Design review of the part built by this model. Coordinates are the model's own, in mm. Face numbers are marked on the shaded views. A direction names the side the tool comes from. Give positions to 0.01 mm unless a question says otherwise; leave off trailing zeros. Loops run counter-clockwise (first coordinate to the right, second up) from the corner with the lowest first, then second, coordinate; pieces in that order, holes last.
from build123d import *

# Parameters (mm, degrees)
SKETCH030_W             = 25
SKETCH030_H             = 15
PAD007_DEPTH            = 2
PAD008_DEPTH            = 7.5
SKETCH032_R             = 1.5
POCKET007_DEPTH         = 7.25
SKETCH031_R             = 1.75
POCKET008_DEPTH         = 5
PAD009_DEPTH            = 2
CHAMFER005_SIZE         = 1
SKETCH035_R             = 2.125
SKETCH035_R_2           = 1.75
PAD010_DEPTH            = 1.1
BODY003_PLACEMENT_ANGLE = 180


with BuildPart() as part:
    # Sketch030 → Pad007 (new body)
    with BuildSketch(Plane.YZ):
        Rectangle(SKETCH030_W, SKETCH030_H)
    extrude(amount=PAD007_DEPTH)

    # Sketch033 (on Face4 of Pad007) → Pad008 (join)
    with BuildSketch(Plane(origin=(0, 0, 7.5), x_dir=(0, -1, 0), z_dir=(0, 0, 1))):
        Polygon((-15, -23.23103), (15, -23.23103), (17, -9.88), (15, 2), (-15, 2), (-17, -9.88), align=None)
    extrude(amount=PAD008_DEPTH)

    # Sketch032 (on Face13 of Pad008) → Pocket007 (cut)
    with BuildSketch(Plane(origin=(0, 0, 15), x_dir=(0, -1, 0), z_dir=(0, 0, 1))):
        with Locations((11.75, -2.18)):
            Circle(SKETCH032_R)
        with Locations((-11.75, -2.18)):
            Circle(SKETCH032_R)
    extrude(amount=-POCKET007_DEPTH, mode=Mode.SUBTRACT)

    # Sketch031 (on Face4 of Pad008) → Pocket008 (cut)
    with BuildSketch(Plane(origin=(0, 0, 0), x_dir=(0, 1, 0), z_dir=(-1, 0, 0))):
        with Locations((-6.925, 0)):
            Circle(SKETCH031_R)
        with Locations((6.925, 0)):
            Circle(SKETCH031_R)
    extrude(amount=-POCKET008_DEPTH, mode=Mode.SUBTRACT)

    # Sketch034 (on Face1 of Pocket008) → Pad009 (join)
    with BuildSketch(Plane(origin=(0, -12.5, 0), x_dir=(0, 0, -1), z_dir=(0, -1, 0))):
        Polygon((-7.5, -9.88), (7.5, 0), (-7.5, 0), align=None)
    pad009 = extrude(amount=-PAD009_DEPTH)

    # Mirrored001: Pad009 across XZ
    add(pad009.mirror(Plane.XZ))

    # Chamfer005
    chamfer005_edges = [part.edges().sort_by_distance(p)[0] for p in [
        (-2.18, 13.25, 15),
        (-2.18, -10.25, 15),
    ]]
    chamfer(chamfer005_edges, length=CHAMFER005_SIZE)

    # Sketch035 (on Face19 of Chamfer005) → Pad010 (join, symmetric)
    with BuildSketch(Plane(origin=(1, 0, 0), x_dir=(0, 1, 0), z_dir=(-1, 0, 0))):
        with Locations((-6.925, 0)):
            Circle(SKETCH035_R)
        with Locations((-6.925, 0)):
            Circle(SKETCH035_R_2, mode=Mode.SUBTRACT)
        with Locations((6.925, 0)):
            Circle(SKETCH035_R)
        with Locations((6.925, 0)):
            Circle(SKETCH035_R_2, mode=Mode.SUBTRACT)
    extrude(amount=PAD010_DEPTH, both=True)


with BuildPart() as part_1:
    # Body003 placement: moved
    add(part.part.rotate(Axis((0, 0, 0), (1, 0, 0)), BODY003_PLACEMENT_ANGLE))


solid = part_1.part
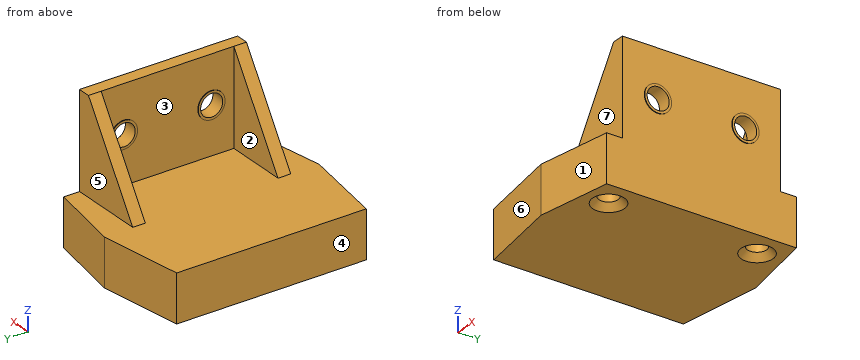
Q1. Tool access review of the marked faces 5, 6 and 7: name each direction out of +Z, -Z, +X, -X, +Y, -Y from which nothing blocks a thin tool from reaching the whole face with its end or side.
Results:
face 5: +Z, +X, -X, +Y
face 6: +Z, -Z, -X, -Y
face 7: +Z, +X, -X, -Y
Q2. Draft analysis for pull direction Y (two halves, no side actions). For the marked faces 1, 2, 3 and 4, state which applies: pulls with the +Y half, pulls with the -Y half, needs draft (parallel to the pull), parting line crosses it, or undercut.
Results:
face 1: pulls with the -Y half
face 2: undercut
face 3: undercut
face 4: needs draft
Q3. Take a section at B-B (z = 0). Give the number of separate pieces and of enclosed holes in the cut face, plus the area to 3 significant figures.
Results:
separate pieces: 3
enclosed holes: 0
area: 56.1 mm2
Q4. Insertion check: pin 1 (4 mm diameter, centred on y = -6.925, z = 0, fed in from -X); pin 2 (3 mm diameter, centred on y = -13, z = 2.5, fed in from -X); pin 3 (11 mm diameter, centred on x = -5, z = -1, fed in from +Y); pin 4 (1.5 mm diameter, centred on y = -13.5, z = -6, fed in from +X). Each pin has a flat end and moves straight along its axis. Give the tip position at first contact, or say it passes through.
Results:
pin 1: stops at x = -0.1
pin 2: stops at x = -4.22
pin 3: stops at y = 12.5
pin 4: passes through
Q5. Take a section at D-D (x = -2.18). Give the boundary of the cut face in (y, z), plus the area to 3 significant figures.
Results:
outline: (-15.7, -15) - (-14.25, -15) - (-13.25, -14) - (-13.25, -7.75) - (-10.25, -7.75) - (-10.25, -14) - (-9.25, -15) - (9.25, -15) - (10.25, -14) - (10.25, -7.75) - (13.25, -7.75) - (13.25, -14) - (14.25, -15) - (15.7, -15) - (15.7, -7.5) - (12.5, -7.5) - (12.5, 4.19) - (10.5, 4.19) - (10.5, -7.5) - (-10.5, -7.5) - (-10.5, 4.19) - (-12.5, 4.19) - (-12.5, -7.5) - (-15.7, -7.5) - close
area: 237 mm2
Q6. Take a section at C-C (z = -13). Give the boundary of the cut face in (x, y), plus the area to 3 significant figures.
Results:
outline: (-23.23, -15) - (-9.88, -17) - (2, -15) - (2, 15) - (-9.88, 17) - (-23.23, 15) - close; hole circle Ø3 at (-2.18, -11.75); hole circle Ø3 at (-2.18, 11.75)
area: 793 mm2
Q7. Take a section at A-A (y = 11.75). Give the boundary of the cut face in (x, z).
Results:
outline: (-23.23, -15) - (-4.68, -15) - (-3.68, -14) - (-3.68, -7.75) - (-0.68, -7.75) - (-0.68, -14) - (0.32, -15) - (2, -15) - (2, 7.5) - (0, 7.5) - (-9.88, -7.5) - (-23.23, -7.5) - close
Q8. Wall thickness on line 1 (Y direction, x = -1.5, z = -2.5); line 2 (Z direction, x = -18.75, y = 2.5); line 3 (X direction, y = -4.5, z = -4.5): over which ranges is each line inside the solid? List them lowest first.
Results:
line 1: y = -12.5 to -10.5, 10.5 to 12.5
line 2: z = -15 to -7.5
line 3: x = 0 to 2
